For this review, use the dimensioned drawing (mm, ordinates from the lowest corner) and the shaded views. Give positions to 0.01 mm unless a question says otherwise; leave off trailing zeros. Write each loop counter-clockwise with the first axis right and the second up, starting at its lowest first coordinate (ties: lowest second). Pieces come first, ordered by that corner, then holes. Notation, with made-up numbers: (7.25, -19) -> (54.25, -19) arc R14 cw to (54.25, -1) -> close; hole circle Ø9 at (57, -20). An arc over 180 degrees is marked (long way). Return JSON: item names as keys, results as strings.
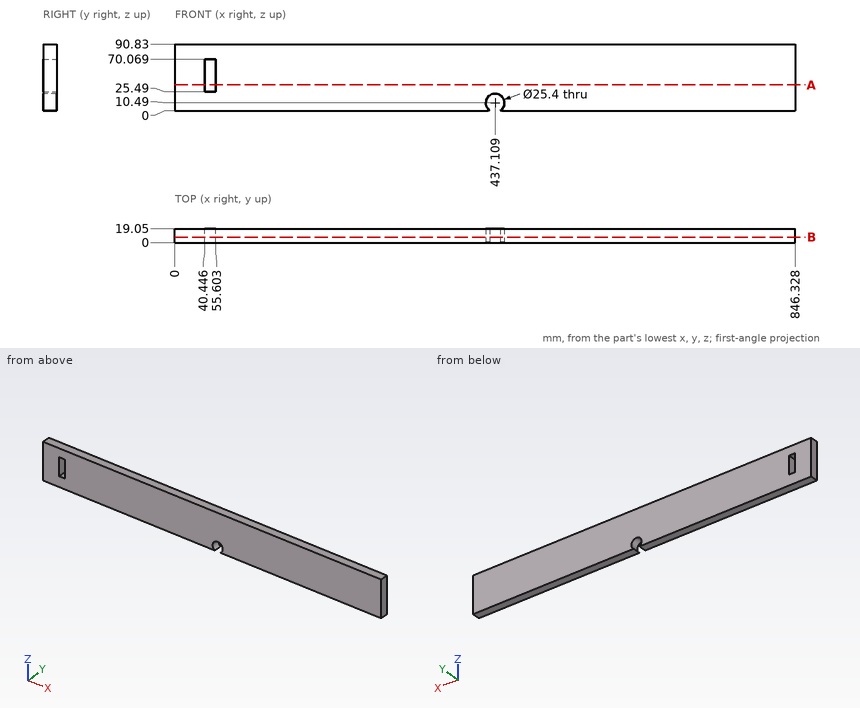
1. To check wall thickness, follow probe 1 along Z at (x, y) = (51, 6); probe 2 along X at (y, z) = (15.25, 43); probe 3 along Z at (x, y) = (427.5, 17.5) (1 decimal). State the ranges of each line that lie inside material, in increasing order.
Results found:
{"probe 1": "z = 0 to 25.49, 70.07 to 90.83", "probe 2": "x = 0 to 40.45, 55.6 to 846.33", "probe 3": "z = 0 to 2.2, 18.8 to 90.8"}
2. Add section A-A, the plane z = 35. State the section outline as (x, y) points, plus the area to 3 significant figures.
Results found:
{"outline": "(0, 0) -> (40.45, 0) -> (40.45, 19.05) -> (0, 19.05) -> close; (55.6, 0) -> (846.33, 0) -> (846.33, 19.05) -> (55.6, 19.05) -> close", "area": "15,800 mm²"}
3. For pin 1 (9.5 mm diameter, centred on y = 9, z = 40, fed in from -X); pin 2 (15 mm diameter, centred on x = 437.11, z = 10.49, fed in from +Y), all flat-tipped, find the tip position at first contact; note any pin that passes through.
Results found:
{"pin 1": "stops at x = 0", "pin 2": "passes through"}
4. Add section B-B, the plane y = 7.25. State the section outline as (x, z) points.
Results found:
{"outline": "(0, 0) -> (429.95, 0) arc R12.7 cw (long way) to (444.27, 0) -> (846.33, 0) -> (846.33, 90.83) -> (0, 90.83) -> close; hole (40.45, 25.49) -> (55.6, 25.49) -> (55.6, 70.07) -> (40.45, 70.07) -> close"}
